```python
from build123d import *

# Parameters (mm, degrees)
SKETCH1_W                       = 45
SKETCH1_H                       = 200
BOSS_EXTRUDE1_DEPTH             = 1700
FILLET1_R                       = 4
SKETCH9_R                       = 30
CUT_EXTRUDE1_DEPTH              = 50
SKETCH10_R                      = 5.5
CUT_EXTRUDE2_DEPTH              = 50
SKETCH11_R                      = 5.5
CUT_EXTRUDE3_DEPTH              = 50
SKETCH12_R                      = 5.5
CUT_EXTRUDE4_DEPTH              = 50
SKETCH13_R                      = 5.5
CUT_EXTRUDE5_DEPTH              = 50
SKETCH14_R                      = 5.5
CUT_EXTRUDE6_DEPTH              = 50
SKETCH15_R                      = 5.5
CUT_EXTRUDE7_DEPTH              = 50
SKETCH16_R                      = 18
CUT_EXTRUDE8_DEPTH              = 30
F_6_0MM_DOWEL_SLOT_D            = 6
F_6_0MM_DOWEL_SLOT_DEPTH        = 128.197418143
F_6_0MM_DOWEL_SLOT_CSINK_D      = 6.05
F_6_0MM_DOWEL_SLOT_CSINK_ANGLE  = 90
F_6_0MM_DOWEL_SLOT_TIP          = 1.802581857
F_6_0MM_DOWEL_SLOT1_D           = 6
F_6_0MM_DOWEL_SLOT1_DEPTH       = 63.197418143
F_6_0MM_DOWEL_SLOT1_CSINK_D     = 6.05
F_6_0MM_DOWEL_SLOT1_CSINK_ANGLE = 90
F_6_0MM_DOWEL_SLOT1_TIP         = 1.802581857
SKETCH25_R                      = 18
CUT_EXTRUDE9_DEPTH              = 30
F_6_0MM_DOWEL_SLOT2_D           = 6
F_6_0MM_DOWEL_SLOT2_DEPTH       = 48.197418143
F_6_0MM_DOWEL_SLOT2_CSINK_D     = 6.05
F_6_0MM_DOWEL_SLOT2_CSINK_ANGLE = 90
F_6_0MM_DOWEL_SLOT2_TIP         = 1.802581857
F_8_0MM_DOWEL_SLOT4_D           = 8
F_8_0MM_DOWEL_SLOT4_DEPTH       = 137.596557524
F_8_0MM_DOWEL_SLOT4_CSINK_D     = 8.05
F_8_0MM_DOWEL_SLOT4_CSINK_ANGLE = 90
F_8_0MM_DOWEL_SLOT4_TIP         = 2.403442476


with BuildPart() as part:
    # Sketch1 → Boss-Extrude1 (new body)
    with BuildSketch(Plane.XY):
        with Locations((-8.688255411, 34.272684877)):
            Rectangle(SKETCH1_W, SKETCH1_H)
    extrude(amount=BOSS_EXTRUDE1_DEPTH)

    # Fillet1
    fillet1_edges = [part.edges().sort_by_distance(p)[0] for p in [
        (13.811744589, 134.272684877, 850),
        (13.811744589, -65.727315123, 850),
        (-31.188255411, -65.727315123, 850),
        (-31.188255411, 134.272684877, 850),
    ]]
    fillet(fillet1_edges, radius=FILLET1_R)

    # Sketch9 → Cut-Extrude1 (cut)
    with BuildSketch(Plane(origin=(13.811744589, 0, 0), x_dir=(0, 0, -1), z_dir=(1, 0, 0))):
        with Locations((-1337, -5.727315122)):
            Circle(SKETCH9_R)
    extrude(amount=-CUT_EXTRUDE1_DEPTH, mode=Mode.SUBTRACT)

    # Sketch10 → Cut-Extrude2 (cut)
    with BuildSketch(Plane(origin=(13.811744589, 0, 0), x_dir=(0, 0, -1), z_dir=(1, 0, 0))):
        with Locations((-1392, 97.272684878)):
            Circle(SKETCH10_R)
    extrude(amount=-CUT_EXTRUDE2_DEPTH, mode=Mode.SUBTRACT)

    # Sketch11 → Cut-Extrude3 (cut)
    with BuildSketch(Plane(origin=(13.811744589, 0, 0), x_dir=(0, 0, -1), z_dir=(1, 0, 0))):
        with Locations((-1392, -33.727315122)):
            Circle(SKETCH11_R)
    extrude(amount=-CUT_EXTRUDE3_DEPTH, mode=Mode.SUBTRACT)

    # Sketch12 → Cut-Extrude4 (cut)
    with BuildSketch(Plane(origin=(13.811744589, 0, 0), x_dir=(0, 0, -1), z_dir=(1, 0, 0))):
        with Locations((-1217, 97.272684878)):
            Circle(SKETCH12_R)
    extrude(amount=-CUT_EXTRUDE4_DEPTH, mode=Mode.SUBTRACT)

    # Sketch13 → Cut-Extrude5 (cut)
    with BuildSketch(Plane(origin=(13.811744589, 0, 0), x_dir=(0, 0, -1), z_dir=(1, 0, 0))):
        with Locations((-1217, -33.727315122)):
            Circle(SKETCH13_R)
    extrude(amount=-CUT_EXTRUDE5_DEPTH, mode=Mode.SUBTRACT)

    # Sketch14 → Cut-Extrude6 (cut)
    with BuildSketch(Plane(origin=(13.811744589, 0, 0), x_dir=(0, 0, -1), z_dir=(1, 0, 0))):
        with Locations((-1042, -33.727315122)):
            Circle(SKETCH14_R)
    extrude(amount=-CUT_EXTRUDE6_DEPTH, mode=Mode.SUBTRACT)

    # Sketch15 → Cut-Extrude7 (cut)
    with BuildSketch(Plane(origin=(13.811744589, 0, 0), x_dir=(0, 0, -1), z_dir=(1, 0, 0))):
        with Locations((-1042, 97.272684878)):
            Circle(SKETCH15_R)
    extrude(amount=-CUT_EXTRUDE7_DEPTH, mode=Mode.SUBTRACT)

    # Sketch16 → Cut-Extrude8 (cut)
    with BuildSketch(Plane.ZY.offset(31.188255411)):
        with Locations(Location((50, -25.727315123, 0), (0, 0, 270))):
            Circle(SKETCH16_R)
        with Locations(Location((50, 34.272684877, 0), (0, 0, 270))):
            Circle(SKETCH16_R)
        with Locations(Location((50, 91.272684877, 0), (0, 0, 270))):
            Circle(SKETCH16_R)
    extrude(amount=-CUT_EXTRUDE8_DEPTH, mode=Mode.SUBTRACT)

    # Ø6.0mm Dowel Slot
    with Locations(Plane(origin=(-854.153391206, -65.727315123, 36.0493232), x_dir=(0.6427592920058945, 7.226860248094423e-15, 0.7660682035824756), z_dir=(-0.7660682035824756, -8.613283256507993e-15, 0.6427592920058945))):
        with Locations((1247.849951753, 160), (1247.849951753, 100), (1247.849951753, 40)):
            CounterSinkHole(F_6_0MM_DOWEL_SLOT_D / 2, F_6_0MM_DOWEL_SLOT_CSINK_D / 2, depth=F_6_0MM_DOWEL_SLOT_DEPTH, counter_sink_angle=F_6_0MM_DOWEL_SLOT_CSINK_ANGLE)
            with Locations((0, 0, -(F_6_0MM_DOWEL_SLOT_DEPTH + F_6_0MM_DOWEL_SLOT_TIP / 2))):  # 118° drill point
                Cone(0, F_6_0MM_DOWEL_SLOT_D / 2, F_6_0MM_DOWEL_SLOT_TIP, mode=Mode.SUBTRACT)

    # Ø6.0mm Dowel Slot1
    with Locations(Plane(origin=(13.811744589, -65.727315123, 0), x_dir=(0, 0, -1), z_dir=(1, 0, 0))):
        with Locations((-872.5, 160), (-872.5, 100), (-872.5, 40)):
            CounterSinkHole(F_6_0MM_DOWEL_SLOT1_D / 2, F_6_0MM_DOWEL_SLOT1_CSINK_D / 2, depth=F_6_0MM_DOWEL_SLOT1_DEPTH, counter_sink_angle=F_6_0MM_DOWEL_SLOT1_CSINK_ANGLE)
            with Locations((0, 0, -(F_6_0MM_DOWEL_SLOT1_DEPTH + F_6_0MM_DOWEL_SLOT1_TIP / 2))):  # 118° drill point
                Cone(0, F_6_0MM_DOWEL_SLOT1_D / 2, F_6_0MM_DOWEL_SLOT1_TIP, mode=Mode.SUBTRACT)

    # Sketch25 → Cut-Extrude9 (cut)
    with BuildSketch(Plane.ZY.offset(31.188255411)):
        with Locations(Location((1650, 94.272684877, 0), (0, 0, 270))):
            Circle(SKETCH25_R)
        with Locations(Location((1650, -25.727315123, 0), (0, 0, 270))):
            Circle(SKETCH25_R)
    extrude(amount=-CUT_EXTRUDE9_DEPTH, mode=Mode.SUBTRACT)

    # Ø6.0mm Dowel Slot2
    with Locations(Plane(origin=(-811.188255411, -65.727315123, 1700), x_dir=(1, 0, 0), z_dir=(0, 0, 1))):
        with Locations((25, 160), (25, 40), (800, 160), (800, 40)):
            CounterSinkHole(F_6_0MM_DOWEL_SLOT2_D / 2, F_6_0MM_DOWEL_SLOT2_CSINK_D / 2, depth=F_6_0MM_DOWEL_SLOT2_DEPTH, counter_sink_angle=F_6_0MM_DOWEL_SLOT2_CSINK_ANGLE)
            with Locations((0, 0, -(F_6_0MM_DOWEL_SLOT2_DEPTH + F_6_0MM_DOWEL_SLOT2_TIP / 2))):  # 118° drill point
                Cone(0, F_6_0MM_DOWEL_SLOT2_D / 2, F_6_0MM_DOWEL_SLOT2_TIP, mode=Mode.SUBTRACT)

    # Ø8.0mm Dowel Slot4
    with Locations(Plane(origin=(-811.188255411, -65.727315123, -90), x_dir=(-1, 0, 0), z_dir=(0, 0, -1))):
        with Locations((-802.5, 40), (-802.5, 100), (-802.5, 157)):
            CounterSinkHole(F_8_0MM_DOWEL_SLOT4_D / 2, F_8_0MM_DOWEL_SLOT4_CSINK_D / 2, depth=F_8_0MM_DOWEL_SLOT4_DEPTH, counter_sink_angle=F_8_0MM_DOWEL_SLOT4_CSINK_ANGLE)
            with Locations((0, 0, -(F_8_0MM_DOWEL_SLOT4_DEPTH + F_8_0MM_DOWEL_SLOT4_TIP / 2))):  # 118° drill point
                Cone(0, F_8_0MM_DOWEL_SLOT4_D / 2, F_8_0MM_DOWEL_SLOT4_TIP, mode=Mode.SUBTRACT)


solid = part.part
```
CAD build for the part. Positions are in the model's coordinates, mm. A direction names the side the tool comes from. Give positions to 0.01 mm unless a question says otherwise; leave off trailing zeros. Loops run counter-clockwise (first coordinate to the right, second up) from the corner with the lowest first, then second, coordinate; pieces in that order, holes last. Notation, with made-up numbers: (-39.5, 56) - (-10.5, 56) arc R25 ccw to (-10.5, 73) - close; hole circle Ø5 at (49, -27.5). An arc over 180 degrees is marked (long way). Put each result on its own line as item: value.
Q1. Slice it at B-B (z = 50). Give the cut face in (x, y).
Filled in:
outline: (-31.19, -61.73) arc R4 ccw to (-27.19, -65.73) - (9.81, -65.73) arc R4 ccw to (13.81, -61.73) - (13.81, 130.27) arc R4 ccw to (9.81, 134.27) - (-27.19, 134.27) arc R4 ccw to (-31.19, 130.27) - (-31.19, 109.27) - (-1.19, 109.27) - (-1.19, 73.27) - (-31.19, 73.27) - (-31.19, 52.27) - (-1.19, 52.27) - (-1.19, 16.27) - (-31.19, 16.27) - (-31.19, -7.73) - (-1.19, -7.73) - (-1.19, -43.73) - (-31.19, -43.73) - close
Q2. Mould opens along Y. For faces 1 (the face through (-9, -65.727, 838)), 2 (the face through (-10.17, 93.12, 953.2)), 3 (the face through (-16.4, 74.1, 55.4)), 4 (the face through (-14, 36, 0)) say: pulls with the +Y half, pulls with the -Y half, needs draft (parallel to the pull), parting line crosses it, or undercut.
Filled in:
face 1: pulls with the -Y half
face 2: undercut
face 3: undercut
face 4: needs draft
Q3. Slice it at C-C (z = 1650). Give the cut face in (x, y).
Filled in:
outline: (-31.19, -61.73) arc R4 ccw to (-27.19, -65.73) - (9.81, -65.73) arc R4 ccw to (13.81, -61.73) - (13.81, 130.27) arc R4 ccw to (9.81, 134.27) - (-27.19, 134.27) arc R4 ccw to (-31.19, 130.27) - (-31.19, 112.27) - (-1.19, 112.27) - (-1.19, 76.27) - (-31.19, 76.27) - (-31.19, -7.73) - (-1.19, -7.73) - (-1.19, -43.73) - (-31.19, -43.73) - close
Q4. Flat gauge pins, fed straight in: pin 1 (21.5 mm diameter, centred on y = -25.73, z = 1650, fed in from -X); pin 2 (6.5 mm diameter, centred on x = -8.69, y = 34.27, fed in from -Z). Where does each tip first touch, or does it go through?
Filled in:
pin 1: stops at x = -1.19
pin 2: stops at z = 67.7
Q5. Tool access for faces 5 (the face through (-16.398, 98.175, 1632.428)), 6 (the face through (-9, 134.273, 838)): list every direction of +Z, -Z, +X, -X, +Y, -Y with a clear straight run to the whole face (end or side of a thin tool).
Filled in:
face 5: -X
face 6: +Z, -Z, +X, -X, +Y
Q6. Slice it at A-A (z = 1337). Give the cut face in (x, y).
Filled in:
outline: (-31.19, -61.73) arc R4 ccw to (-27.19, -65.73) - (9.81, -65.73) arc R4 ccw to (13.81, -61.73) - (13.81, -35.73) - (-31.19, -35.73) - close; (-31.19, 24.27) - (13.81, 24.27) - (13.81, 130.27) arc R4 ccw to (9.81, 134.27) - (-27.19, 134.27) arc R4 ccw to (-31.19, 130.27) - close
Q7. Probe line 1 along Y through (x, z) = (-11.5, 872.5); line 2 along Z through (x, y) = (-16, -7.5); line 3 along Z through (x, y) = (-19, 32). List the from-to ranges inside material, lowest first.
Filled in:
line 1: y = -65.73 to -28.73, -22.73 to 31.27, 37.27 to 91.27, 97.27 to 134.27
line 2: z = 0 to 1307.05, 1366.95 to 1700
line 3: z = 0 to 32.14, 67.86 to 870.54, 874.46 to 961.67, 966.78 to 1700
